```python
from build123d import *

# Parameters (mm, degrees)
SKETCH1_W           = 100
SKETCH1_H           = 40
BOSS_EXTRUDE1_DEPTH = 30
SKETCH2_W           = 50
SKETCH2_H           = 20
CUT_EXTRUDE1_DEPTH  = 30
SKETCH3_W           = 60
SKETCH3_H           = 10
CUT_EXTRUDE3_DEPTH  = 110
BOSS_EXTRUDE2_DEPTH = 10
SKETCH5_W           = 100
SKETCH5_H           = 10
BOSS_EXTRUDE3_DEPTH = 10
CUT_EXTRUDE4_DEPTH  = 45
SKETCH7_W           = 100
SKETCH7_H           = 130
BOSS_EXTRUDE4_DEPTH = 20
SKETCH8_R           = 30
CUT_EXTRUDE5_DEPTH  = 20
CUT_EXTRUDE6_DEPTH  = 20
BOSS_EXTRUDE5_DEPTH = 10
SKETCH12_W          = 60
SKETCH12_H          = 10
CUT_EXTRUDE9_DEPTH  = 56


with BuildPart() as part:
    # Sketch1 → Boss-Extrude1 (new body)
    with BuildSketch(Plane.XY):
        with Locations((50, 20)):
            Rectangle(SKETCH1_W, SKETCH1_H)
    extrude(amount=BOSS_EXTRUDE1_DEPTH)

    # Sketch2 → Cut-Extrude1 (cut)
    with BuildSketch(Plane.XY.offset(30)):
        with Locations((25, 10)):
            Rectangle(SKETCH2_W, SKETCH2_H)
    extrude(amount=-CUT_EXTRUDE1_DEPTH, mode=Mode.SUBTRACT)

    # Sketch3 → Cut-Extrude3 (cut)
    with BuildSketch(Plane(origin=(0, 40, 0), x_dir=(1, 0, 0), z_dir=(0, 1, 0))):
        with Locations((50, -5)):
            Rectangle(SKETCH3_W, SKETCH3_H)
    extrude(amount=-CUT_EXTRUDE3_DEPTH, mode=Mode.SUBTRACT)

    # Sketch4 → Boss-Extrude2 (add)
    with BuildSketch(Plane(origin=(0, 40, 0), x_dir=(1, 0, 0), z_dir=(0, 1, 0))):
        Polygon((100, 0), (100, -30), (0, -30), (0, 0), (20, 0), (20, -10), (80, -10), (80, 0), align=None)
    extrude(amount=BOSS_EXTRUDE2_DEPTH)

    # Sketch5 → Boss-Extrude3 (add)
    with BuildSketch(Plane.XY.offset(30)):
        with Locations((50, 45)):
            Rectangle(SKETCH5_W, SKETCH5_H)
    extrude(amount=BOSS_EXTRUDE3_DEPTH)

    # Sketch6 → Cut-Extrude4 (cut)
    with BuildSketch(Plane(origin=(0, 50, 0), x_dir=(1, 0, 0), z_dir=(0, 1, 0))):
        Polygon((0, -10), (30, -40), (0, -40), align=None)
    extrude(amount=-CUT_EXTRUDE4_DEPTH, mode=Mode.SUBTRACT)

    # Sketch7 → Boss-Extrude4 (add)
    with BuildSketch(Plane(origin=(0, 50, 0), x_dir=(1, 0, 0), z_dir=(0, 1, 0))):
        with Locations((50, -65)):
            Rectangle(SKETCH7_W, SKETCH7_H)
    extrude(amount=BOSS_EXTRUDE4_DEPTH)

    # Sketch8 → Cut-Extrude5 (cut)
    with BuildSketch(Plane.XZ.offset(-50)):
        with Locations(Location((50, 80, 0), (0, 0, 270))):
            Circle(SKETCH8_R)
    extrude(amount=-CUT_EXTRUDE5_DEPTH, mode=Mode.SUBTRACT)

    # Sketch9 → Cut-Extrude6 (cut)
    with BuildSketch(Plane(origin=(0, 50, 0), x_dir=(-1, 0, 0), z_dir=(0, -1, 0))):
        with BuildLine():
            Line((0, -130), (0, -80))
            ThreePointArc((0, -80), (-14.644660941, -115.355339059), (-50, -130))
            Line((-50, -130), (0, -130))
        make_face()
        with BuildLine():
            Line((-100, -130), (-50, -130))
            ThreePointArc((-50, -130), (-85.355339059, -115.355339059), (-100, -80))
            Line((-100, -80), (-100, -130))
        make_face()
    extrude(amount=-CUT_EXTRUDE6_DEPTH, mode=Mode.SUBTRACT)

    # Sketch10 → Boss-Extrude5 (add)
    with BuildSketch(Plane(origin=(0, 50, 0), x_dir=(-1, 0, 0), z_dir=(0, -1, 0))):
        with BuildLine():
            Line((-50, -110), (-50, -130))
            ThreePointArc((-50, -130), (-85.355339059, -115.355339059), (-100, -80))
            Line((-100, -80), (-100, -40))
            Line((-100, -40), (-50, -40))
            Line((-50, -40), (-50, -50))
            ThreePointArc((-50, -50), (-80, -80), (-50, -110))
        make_face()
    extrude(amount=BOSS_EXTRUDE5_DEPTH)

    # Sketch12 → Cut-Extrude9 (cut)
    with BuildSketch(Plane.XZ.offset(-50)):
        with Locations((50, 5)):
            Rectangle(SKETCH12_W, SKETCH12_H)
    extrude(amount=-CUT_EXTRUDE9_DEPTH, mode=Mode.SUBTRACT)


solid = part.part
```
Could you check a few things on this model? Use its own coordinates, in mm. A direction names the side the tool comes from. Give positions to 0.01 mm unless a question says otherwise; leave off trailing zeros. Order: outer loops, then holes, each group sorted by start corner. A loop starts at its lowest first (then second) coordinate and runs counter-clockwise, first axis right, second up.
Q1. Suppose I cut it at C-C, the plane z = 76.5. Write out the boundary of the cut face in (x, y).
Q2. I'm going to push flat-ended pins straight in: P1, Ø10, axis at x = 53, y = 34.5, coming from the +Z side; P2, Ø11, axis at y = 43.5, z = 124.5, coming from the -X side; P3, Ø11, axis at x = 37, y = 46.5, coming from the +Z side. Where does each tip first touch, or does it pass through?
Q3. For faces 1 (the flat face through (10, 45, 0)), 2 (the flat face through (25, 20, 15)), 3 (the flat face through (69, 20, 30)), 4 (the flat face through (40, 45, 40)), which set-ups out of +Z, -Z, +X, -X, +Y, -Y let a thin tool reach every point of the face, with its end or its side?
Q4. Suppose I cut it at D-D, the plane y = 46. Write out the boundary of the cut face in (x, z).
Q5. If I drill on line 1 along X through (y, z) = (65.75, 80); line 2 along Z through (x, y) = (50, 57.25); line 3 along Y through (x, z) = (95.5, 39), over which ranges is the centre line in solid material (lowest first)?
Q6. Suppose I cut it at B-B, the plane x = 73.5. Write out the boundary of the cut face in (y, z), and give its area (3 significant figures).
Q7. Suppose I cut it at A-A, the plane y = 59. Write out the boundary of the cut face in (x, z).
Solution:
1. outline: (0, 50) - (20.2, 50) - (20.2, 70) - (0, 70) - close; (79.8, 40) - (100, 40) - (100, 70) - (79.8, 70) - close
2. P1: stops at z = 30
2. P2: stops at x = 50
2. P3: stops at z = 129.23
3. face 1: -Z, +X, -X, +Y, -Y
3. face 2: +Z, -Z, -X, -Y
3. face 3: +Z, +X, -X, -Y
3. face 4: +Z, -X, -Y
4. outline: (0, 0) - (20, 0) - (20, 10) - (80, 10) - (80, 0) - (100, 0) - (100, 80) arc R50 ccw to (50, 130) - (50, 110) arc R30 cw to (50, 50) - (50, 40) - (30, 40) - (0, 10) - close
5. line 1: x = 0 to 20, 80 to 100
5. line 2: z = 10 to 50, 110 to 130
5. line 3: y = 40 to 70
6. outline: (0, 10) - (70, 10) - (70, 61.35) - (40, 61.35) - (40, 30) - (0, 30) - close; (40, 98.65) - (70, 98.65) - (70, 124.13) - (40, 124.13) - close
6. area: 3,110 mm2
7. outline: (0, 0) - (20, 0) - (20, 10) - (80, 10) - (80, 0) - (100, 0) - (100, 80) arc R50 ccw to (0, 80) - close; hole circle Ø60 at (50, 80)
